Geometry: see drawing. Coordinates: mm, zero at the bounding-box minimum. Give positions to 0.01 mm unless a question says otherwise; leave off trailing zeros. Loops run counter-clockwise (first coordinate to the right, second up) from the corner with the lowest first, then second, coordinate; pieces in that order, holes last. Notation, with made-up numbers: M 39,86.5 L 84,86.5 A23 cw 84,105.5 Z; hole C -16,-2.5 d3. An arc over 180 degrees is marked long. Put each result on its own line as item: value.
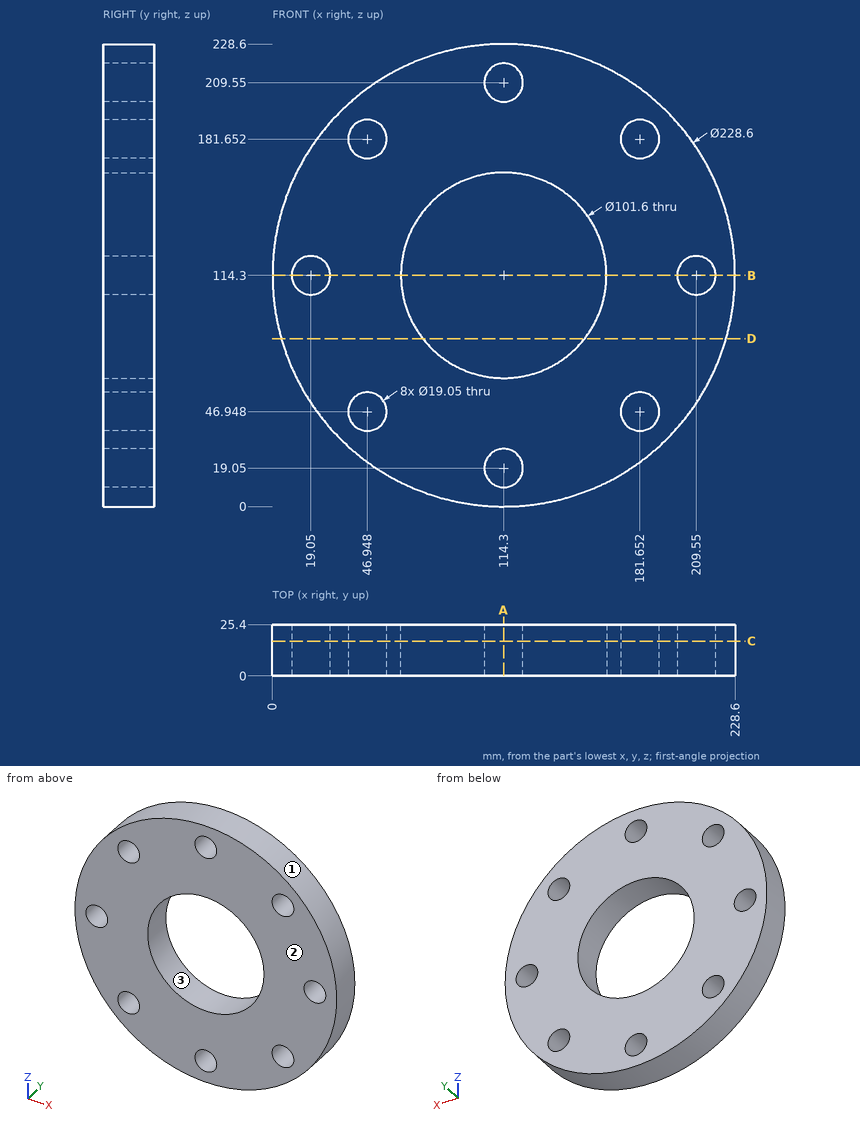
1. Section query B-B (z = 114.3). Output: boundary loops of the cut face in (x, y) (3 decimals).
Found:
outline: M 0,0 L 9.525,0 L 9.525,25.4 L 0,25.4 Z; M 28.575,0 L 63.5,0 L 63.5,25.4 L 28.575,25.4 Z; M 165.1,0 L 200.025,0 L 200.025,25.4 L 165.1,25.4 Z; M 219.075,0 L 228.6,0 L 228.6,25.4 L 219.075,25.4 Z
2. Section query C-C (y = 17.25). State how many separate pieces and enclosed holes the cut face has, plus the area to 3 significant figures.
Found:
separate pieces: 1
enclosed holes: 9
area: 30,700 mm^2
3. Material intervals for line 1 (Z direction, x = 109, y = 5.25); line 2 (X direction, y = 7.25, z = 185) (1 decimal); line 3 (X direction, y = 23.25, z = 46.5), sorted ascending. Write a range as from..to.
Found:
line 1: 0.12..11.14, 26.96..63.78, 164.82..201.64, 217.46..228.48
line 2: 24.5..38, 55.9..172.7, 190.6..204.1
line 3: 22.28..37.43, 56.46..172.14, 191.17..206.32
4. Section query A-A (x = 114.3). Output: boundary loops of the cut face in (y, z) (3 decimals), plus the area to 3 significant figures.
Found:
outline: M 0,0 L 25.4,0 L 25.4,9.525 L 0,9.525 Z; M 0,28.575 L 25.4,28.575 L 25.4,63.5 L 0,63.5 Z; M 0,165.1 L 25.4,165.1 L 25.4,200.025 L 0,200.025 Z; M 0,219.075 L 25.4,219.075 L 25.4,228.6 L 0,228.6 Z
area: 2,260 mm^2
5. Section query D-D (z = 83). Output: boundary loops of the cut face in (x, y), plus the area to 3 significant figures.
Found:
outline: M 4.37,0 L 74.29,0 L 74.29,25.4 L 4.37,25.4 Z; M 154.31,0 L 224.23,0 L 224.23,25.4 L 154.31,25.4 Z
area: 3,550 mm^2
6. Draft query along X for the marked faces 1, 2 and 3. Return one class per face: pulls with the +X half, pulls with the -X half, needs draft (parallel to the pull), parting line crosses it, or undercut.
Found:
face 1: parting line crosses it
face 2: needs draft
face 3: undercut
7. Contact query for flat-ended pins moving along their axis: P1, Ø1.5, axis at y = 8, z = 68.5, coming from the -X side; P2, Ø5, axis at y = 6, z = 57.5, coming from the +X side; P3, Ø6, axis at y = 12.5, z = 24, coming from the +X side. Output: stop coordinate, or through.
Found:
P1: x = 9.25
P2: x = 214.88
P3: x = 188.08
